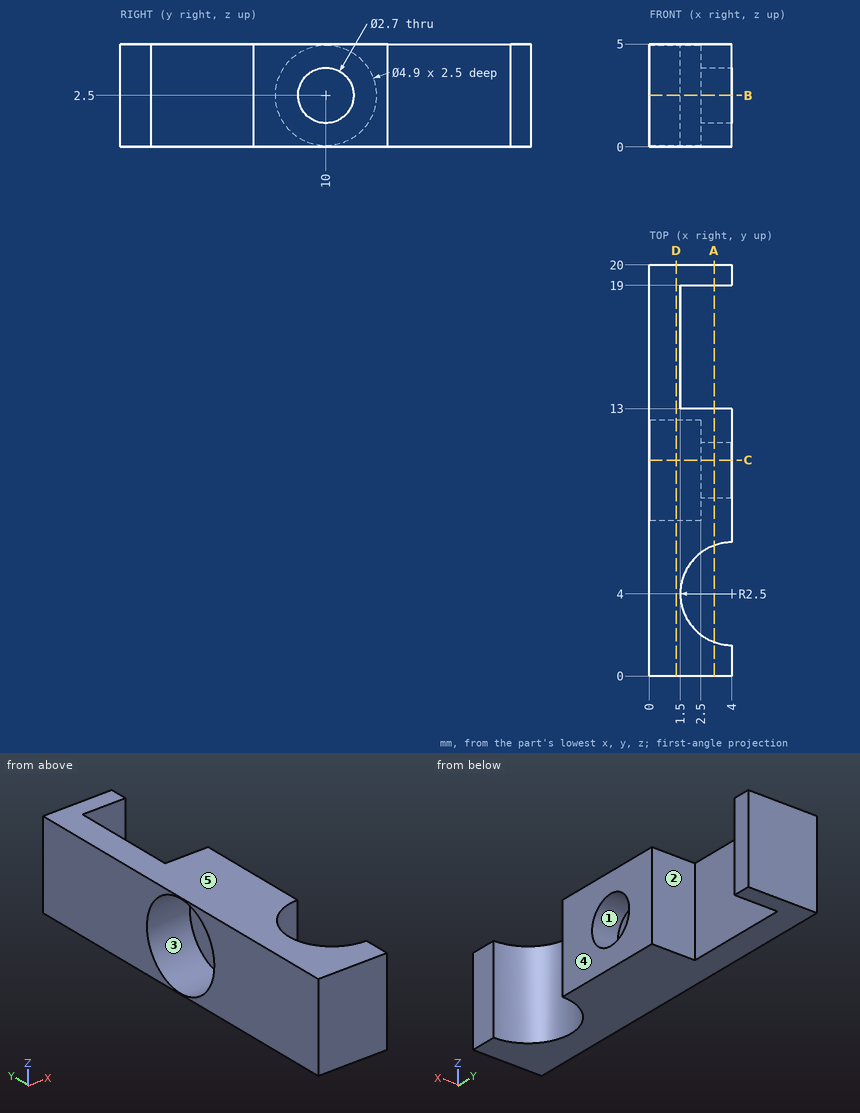
Could you check a few things on this drawing? It's one solid part, dimensions in mm from its lowest x, y, z. A direction names the side the tool comes from. Round coordinates to 2 decimals unless told otherwise and drop trailing zeros. Write each loop counter-clockwise with the first axis right and the second up, starting at its lowest first coordinate (ties: lowest second). Pieces come first, ordered by that corner, then holes. Notation, with made-up numbers: (-22, 7.5) -> (20, 7.5) arc R21 cw to (20, 44.5) -> close; hole circle Ø8 at (85.25, 84.25). An arc over 180 degrees is marked (long way). Use one line per item in the form item = value. Start each with the question number.
Q1. I'm going to push a flat-ended pin straight in: P1, Ø3, axis at y = 10, z = 2.5, coming from the -X side. Where does the tip first touch, or does it pass through?
Q2. Imagine slicing it at C-C (y = 10.5). Please give me the cut outline in (x, z).
Q3. Imagine slicing it at D-D (x = 1.3). Please give me the cut outline in (y, z).
Q4. Imagine slicing it at B-B (z = 2.5). Please give me the cut outline in (x, y).
Q5. If I drill on probe 1 along Y at (x, z) = (2.75, 4.3); probe 2 along Y at (x, z) = (1.85, 2.5); probe 3 along Y at (x, z) = (3.05, 2.45), over which ranges is the centre line in solid material (lowest first)? Write a range as [from, to].
Q6. Imagine slicing it at A-A (x = 3.15). Please give me the cut outline in (y, z), then the cut area to 3 significant figures.
Q7. Which directions (+Z, -Z, +X, -X, +Y, -Y) give clear straight access to the entire face, cutting with the end or side of a thin tool? Please do the marked faces 1 and 2.
Q8. We'd pull the mould along Z, two halves only. Please class the marked faces 3, 4 and 5: +Z half, -Z half, draft (parallel to the pull), parting line (faces both ways), or undercut.
Worked out:
q1.P1 = 2.5
q2.outline = (0, 0) -> (4, 0) -> (4, 1.25) -> (2.5, 1.25) -> (2.5, 0.1) -> (0, 0.1) -> close; (0, 4.9) -> (2.5, 4.9) -> (2.5, 3.75) -> (4, 3.75) -> (4, 5) -> (0, 5) -> close
q3.outline = (0, 0) -> (20, 0) -> (20, 5) -> (0, 5) -> close; hole circle Ø4.9 at (10, 2.5)
q4.outline = (0, 0) -> (4, 0) -> (4, 1.5) arc R2.5 cw to (4, 6.5) -> (4, 8.65) -> (2.5, 8.65) -> (2.5, 7.55) -> (0, 7.55) -> close; (0, 12.45) -> (2.5, 12.45) -> (2.5, 11.35) -> (4, 11.35) -> (4, 13) -> (1.5, 13) -> (1.5, 19) -> (4, 19) -> (4, 20) -> (0, 20) -> close
q5.probe_1 = [0, 1.83], [6.17, 13], [19, 20]
q5.probe_2 = [0, 2.72], [5.28, 7.55], [12.45, 13], [19, 20]
q5.probe_3 = [0, 1.69], [6.31, 8.65], [11.35, 13], [19, 20]
q6.outline = (0, 0) -> (1.65, 0) -> (1.65, 5) -> (0, 5) -> close; (6.35, 0) -> (13, 0) -> (13, 5) -> (6.35, 5) -> close; (19, 0) -> (20, 0) -> (20, 5) -> (19, 5) -> close; hole circle Ø2.7 at (10, 2.5)
q6.area = 40.8 mm^2
q7.face_1 = +X, -X
q7.face_2 = +Z, -Z, +X
q8.face_3 = undercut
q8.face_4 = draft
q8.face_5 = +Z half
